Part model, mm, in its own coordinate system. A direction names the side the tool comes from. Round coordinates to 2 decimals unless told otherwise and drop trailing zeros. Write each loop counter-clockwise with the first axis right and the second up, starting at its lowest first coordinate (ties: lowest second). Pieces come first, ordered by that corner, then holes. Notation, with made-up numbers: (16.25, 49.25) -> (26.25, 49.25) arc R24 cw to (26.25, 85.25) -> close; hole circle Ø9 at (79, 20.5). An arc over 180 degrees is marked (long way). Return JSON: item names as keys, results as strings. Group by question number.
```python
from build123d import *

# Parameters (mm, degrees)
SKETCH1_W          = 95
SKETCH1_H          = 75
MAINSHAPE_DEPTH    = 4.5
SKETCH2_W          = 10
SKETCH2_H          = 9
TAB1_DEPTH         = 4.5
CUT_EXTRUDE2_DEPTH = 64.564927436
SKETCH5_R          = 1.55
SKETCH5_W          = 4.7
SKETCH5_H          = 10.2
CUT_EXTRUDE3_DEPTH = 64.564927436
CUT_EXTRUDE4_DEPTH = 64.564927436
SKETCH8_R          = 1.55
CUT_EXTRUDE6_DEPTH = 64.564927436


with BuildPart() as part:
    # Sketch1 → MainShape (new body)
    with BuildSketch(Plane(origin=(0, 0, 0), x_dir=(1, 0, 0), z_dir=(0, 1, 0))):
        Rectangle(SKETCH1_W, SKETCH1_H)
    extrude(amount=MAINSHAPE_DEPTH)

    # Sketch2 → Tab1 (add, through all)
    with BuildSketch(Plane(origin=(0, 4.5, 0), x_dir=(1, 0, 0), z_dir=(0, 1, 0))):
        with Locations((0, 37.5)):
            Rectangle(SKETCH2_W, SKETCH2_H)
    extrude(amount=-TAB1_DEPTH)

    # Sketch4 → Cut-Extrude2 (cut, through all)
    with BuildSketch(Plane(origin=(0, 4.5, 0), x_dir=(1, 0, 0), z_dir=(0, 1, 0))):
        with BuildLine():
            Line((-38.25, 27), (-41.75, 27))
            Line((-41.75, 27), (-41.75, 29.5))
            Line((-41.75, 29.5), (-42.75, 29.5))
            ThreePointArc((-42.75, 29.5), (-42.926776695, 29.573223305), (-43, 29.75))
            Line((-43, 29.75), (-43, 33.45))
            ThreePointArc((-43, 33.45), (-42.926776695, 33.626776695), (-42.75, 33.7))
            Line((-42.75, 33.7), (-41.75, 33.7))
            Line((-41.75, 33.7), (-41.75, 37.5))
            Line((-41.75, 37.5), (-38.25, 37.5))
            Line((-38.25, 37.5), (-38.25, 33.7))
            Line((-38.25, 33.7), (-37.25, 33.7))
            ThreePointArc((-37.25, 33.7), (-37.073223305, 33.626776695), (-37, 33.45))
            Line((-37, 33.45), (-37, 29.75))
            ThreePointArc((-37, 29.75), (-37.073223305, 29.573223305), (-37.25, 29.5))
            Line((-37.25, 29.5), (-38.25, 29.5))
            Line((-38.25, 29.5), (-38.25, 27))
        make_face()
        with BuildLine():
            Line((38.25, 27), (38.25, 29.5))
            Line((38.25, 29.5), (37.25, 29.5))
            ThreePointArc((37.25, 29.5), (37.073223305, 29.573223305), (37, 29.75))
            Line((37, 29.75), (37, 33.45))
            ThreePointArc((37, 33.45), (37.073223305, 33.626776695), (37.25, 33.7))
            Line((37.25, 33.7), (38.25, 33.7))
            Line((38.25, 33.7), (38.25, 37.5))
            Line((38.25, 37.5), (41.75, 37.5))
            Line((41.75, 37.5), (41.75, 33.7))
            Line((41.75, 33.7), (42.75, 33.7))
            ThreePointArc((42.75, 33.7), (42.926776695, 33.626776695), (43, 33.45))
            Line((43, 33.45), (43, 29.75))
            ThreePointArc((43, 29.75), (42.926776695, 29.573223305), (42.75, 29.5))
            Line((42.75, 29.5), (41.75, 29.5))
            Line((41.75, 29.5), (41.75, 27))
            Line((41.75, 27), (38.25, 27))
        make_face()
    extrude(amount=-CUT_EXTRUDE2_DEPTH, mode=Mode.SUBTRACT)

    # Sketch5 → Cut-Extrude3 (cut, through all)
    with BuildSketch(Plane(origin=(0, 4.5, 0), x_dir=(1, 0, 0), z_dir=(0, 1, 0))):
        with Locations(Location((33, 5, 0), (0, 0, 270))):
            Circle(SKETCH5_R)
        with Locations(Location((-33, 5, 0), (0, 0, 90))):
            Circle(SKETCH5_R)
        with Locations((33, 17.5)):
            Rectangle(SKETCH5_W, SKETCH5_H)
        with Locations((-33, 17.5)):
            Rectangle(SKETCH5_W, SKETCH5_H)
        with Locations((-33, -7.5)):
            Rectangle(SKETCH5_W, SKETCH5_H)
        with Locations((33, -7.5)):
            Rectangle(SKETCH5_W, SKETCH5_H)
    extrude(amount=-CUT_EXTRUDE3_DEPTH, mode=Mode.SUBTRACT)

    # Sketch6 → Cut-Extrude4 (cut, through all)
    with BuildSketch(Plane(origin=(0, 4.5, 0), x_dir=(1, 0, 0), z_dir=(0, 1, 0))):
        with BuildLine():
            Line((-23.5, -14.5), (-23.5, -6.520797289))
            ThreePointArc((-23.5, -6.520797289), (-17.5, 8), (-11.5, -6.520797289))
            Line((-11.5, -6.520797289), (-11.5, -14.5))
            ThreePointArc((-11.5, -14.5), (-17.5, -20.5), (-23.5, -14.5))
        make_face()
    cut_extrude4 = extrude(amount=-CUT_EXTRUDE4_DEPTH, mode=Mode.SUBTRACT)

    # Sketch8 → Cut-Extrude6 (cut, through all)
    with BuildSketch(Plane(origin=(0, 4.5, 0), x_dir=(1, 0, 0), z_dir=(0, 1, 0))):
        with Locations(Location((-38.96, -6.5, 0), (0, 0, 270))):
            Circle(SKETCH8_R)
        with Locations(Location((-38.96, -22.5, 0), (0, 0, 90))):
            Circle(SKETCH8_R)
    cut_extrude6 = extrude(amount=-CUT_EXTRUDE6_DEPTH, mode=Mode.SUBTRACT)

    # Mirror1: Cut-Extrude4, Cut-Extrude6 across plane
    add(cut_extrude4.mirror(Plane(origin=(0, 0, 0), x_dir=(0, 0, 1), z_dir=(1, 0, 0))), mode=Mode.SUBTRACT)
    add(cut_extrude6.mirror(Plane(origin=(0, 0, 0), x_dir=(0, 0, 1), z_dir=(1, 0, 0))), mode=Mode.SUBTRACT)


solid = part.part
```
Item 1: Flat gauge pin, fed straight in: P1, Ø1.3, axis at x = -33.5, y = 3, coming from the -Z side. Where does the tip first touch, or does it go through?
Item 2: Cut at D-D (x = 14.5). Write the cut outline in (y, z), then the cut area to 3 significant figures.
Item 3: Two-plate mould, pull along Z, no slides. Class faces 4 (the face through (33, 2, 2.4)), 5 (the face through (41.75, 2, -36)): released by +Z, released by -Z, zero draft, split by the parting line, or undercut.
Item 4: Cut at C-C (z = -5). Write the cut outline in (x, y), then the cut area to 3 significant figures.
Item 5: Which spindle directions (+Z, -Z, +X, -X, +Y, -Y) get a long thin tool onto all of the face, cutting with end or side? Do faces 1 (the face through (-41.75, 2, -36)), 2 (the face through (35.35, 2, 8)), 3 (the face through (-1, 0, 6)). Say none if no direction does.
Item 6: Cut at A-A (z = 22.5). Write the cut outline in (x, y), then the cut area to 3 significant figures.
Item 7: Cut at B-B (x = 33). Write the cut outline in (y, z), then the cut area to 3 significant figures.
Item 8: Wall check: L1, parallel to Z at x = -33, y = 2.05; L2, parallel to X at y = 3.45, z = 0.5; L3, parallel to X at y = 2.6, z = -14. Give the ranges that are in metal, low to high.
Checks:
{
 "1": {"P1": "stops at z = -37.5"},
 "2": {"outline": "(0, -37.5) -> (4.5, -37.5) -> (4.5, -7.45) -> (0, -7.45) -> close; (0, 19.7) -> (4.5, 19.7) -> (4.5, 37.5) -> (0, 37.5) -> close", "area": "215 mm2"},
 "3": {"face 4": "undercut", "face 5": "zero draft"},
 "4": {"outline": "(-47.5, 0) -> (-34.55, 0) -> (-34.55, 4.5) -> (-47.5, 4.5) -> close; (-31.45, 0) -> (-23.98, 0) -> (-23.98, 4.5) -> (-31.45, 4.5) -> close; (-11.02, 0) -> (11.02, 0) -> (11.02, 4.5) -> (-11.02, 4.5) -> close; (23.98, 0) -> (31.45, 0) -> (31.45, 4.5) -> (23.98, 4.5) -> close; (34.55, 0) -> (47.5, 0) -> (47.5, 4.5) -> (34.55, 4.5) -> close", "area": "283 mm2"},
 "5": {"face 1": "-Z, +Y, -Y", "face 2": "+Y, -Y", "face 3": "+Z, -Z, +X, -X, -Y"},
 "6": {"outline": "(-47.5, 0) -> (-40.51, 0) -> (-40.51, 4.5) -> (-47.5, 4.5) -> close; (-37.41, 0) -> (37.41, 0) -> (37.41, 4.5) -> (-37.41, 4.5) -> close; (40.51, 0) -> (47.5, 0) -> (47.5, 4.5) -> (40.51, 4.5) -> close", "area": "400 mm2"},
 "7": {"outline": "(0, -37.5) -> (4.5, -37.5) -> (4.5, -22.6) -> (0, -22.6) -> close; (0, -12.4) -> (4.5, -12.4) -> (4.5, -6.55) -> (0, -6.55) -> close; (0, -3.45) -> (4.5, -3.45) -> (4.5, 2.4) -> (0, 2.4) -> close; (0, 12.6) -> (4.5, 12.6) -> (4.5, 37.5) -> (0, 37.5) -> close", "area": "232 mm2"},
 "8": {"L1": "z = -37.5 to -22.6, -12.4 to -6.55, -3.45 to 2.4, 12.6 to 37.5", "L2": "x = -47.5 to -26, -9 to 9, 26 to 47.5", "L3": "x = -47.5 to -35.35, -30.65 to 30.65, 35.35 to 47.5"}
}
